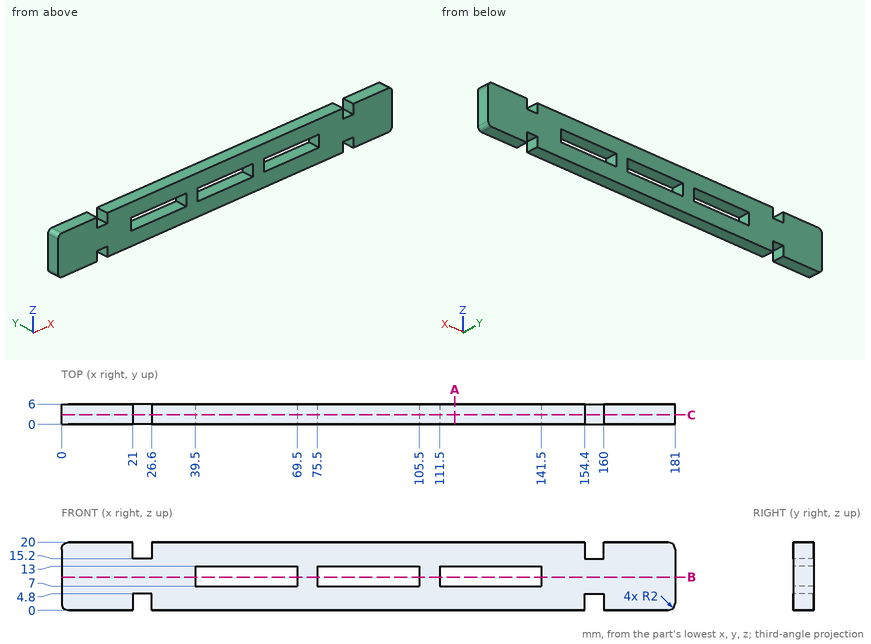
Could you check a few things on this drawing? It's one solid part, dimensions in mm from its lowest x, y, z. Give positions to 0.01 mm unless a question says otherwise; leave off trailing zeros. Write each loop counter-clockwise with the first axis right and the second up, starting at its lowest first coordinate (ties: lowest second). Pieces come first, ordered by that corner, then holes. Notation, with made-up numbers: (-21, -30.5) -> (24, -30.5) arc R15 cw to (24, -7.5) -> close; hole circle Ø11 at (-14, 1.5). An arc over 180 degrees is marked (long way). Answer as CSV lines item,"result". Start each with the question number.
(1) I'm going to push flat-ended pins straight in: pin 1 Ø1.5 at (x, z) = (83.5, 9) entering from +Y; pin 2 Ø1.7 at (x, y) = (23.5, 3.5) entering from -Z. Where does each tip first touch, or does it pass through?
(2) If we section it at B-B, the plane z = 9.75: Write out the boundary of the cut face in (x, y), and give its area (3 significant figures).
(3) If we section it at C-C, the plane y = 2.8: Give the number of separate pieces and of enclosed holes in the cut face, and give its area (3 significant figures).
(4) If we section it at A-A, the plane x = 116: Write out the boundary of the cut face in (y, z), and give its area (3 significant figures).
(5) Please list where these lines run through material, in increasing order: line 1 (X direction, y = 4.5, z = 2.5); line 2 (X direction, y = 0.75, z = 10.5); line 3 (Z direction, x = 138, y = 2.7).
Answer list:
1,pin 1,"through"
1,pin 2,"z = 4.8"
2,outline,"(0, 0) -> (39.5, 0) -> (39.5, 6) -> (0, 6) -> close; (69.5, 0) -> (75.5, 0) -> (75.5, 6) -> (69.5, 6) -> close; (105.5, 0) -> (111.5, 0) -> (111.5, 6) -> (105.5, 6) -> close; (141.5, 0) -> (181, 0) -> (181, 6) -> (141.5, 6) -> close"
2,area,"546 mm^2"
3,separate pieces,"1"
3,enclosed holes,"3"
3,area,"2,970 mm^2"
4,outline,"(0, 0) -> (6, 0) -> (6, 7) -> (0, 7) -> close; (0, 13) -> (6, 13) -> (6, 20) -> (0, 20) -> close"
4,area,"84.0 mm^2"
5,line 1,"0 to 21, 26.6 to 154.4, 160 to 181"
5,line 2,"0 to 39.5, 69.5 to 75.5, 105.5 to 111.5, 141.5 to 181"
5,line 3,"0 to 7, 13 to 20"
